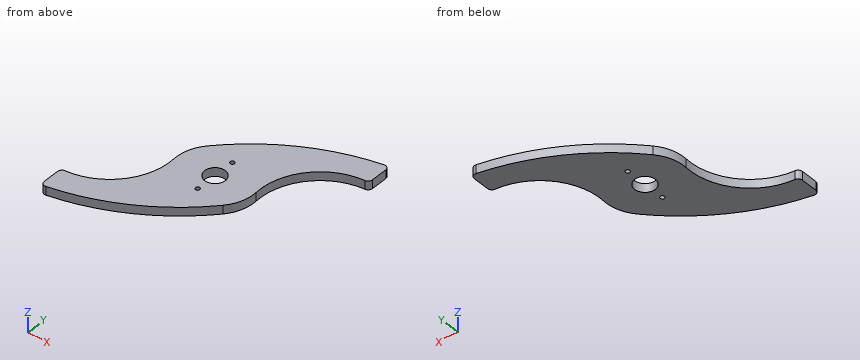
from build123d import *

# Parameters (mm, degrees)
SKETCH1_R           = 45
SKETCH1_R_2         = 12
BOSS_EXTRUDE1_DEPTH = 10
BOSS_EXTRUDE3_START = -10
BOSS_EXTRUDE3_DEPTH = 10
FILLET2_R           = 5
SKETCH3_R           = 2.5
CUT_EXTRUDE1_DEPTH  = 159.845357518


with BuildPart() as part:
    # Sketch1 → Boss-Extrude1 (new body)
    with BuildSketch(Plane.XY):
        Circle(SKETCH1_R)
        Circle(SKETCH1_R_2, mode=Mode.SUBTRACT)
    extrude(amount=BOSS_EXTRUDE1_DEPTH)

    # Sketch2 → Boss-Extrude3 (add)
    with BuildSketch(Plane.XY.offset(10).offset(BOSS_EXTRUDE3_START)):
        with BuildLine():
            ThreePointArc((33.436200174, -30.116781334), (-14.286491123, -42.671960013), (-44.829498519, -3.91357414))
            ThreePointArc((-44.829498519, -3.91357414), (-63.106761283, -57.457908747), (-115, -80))
            Line((-115, -80), (-115, -110))
            ThreePointArc((-115, -110), (-33.84606429, -82.946317595), (33.436200174, -30.116781334))
        make_face()
        with BuildLine():
            Line((115, 80), (115, 110))
            ThreePointArc((115, 110), (33.84606429, 82.946317595), (-33.436200174, 30.116781334))
            ThreePointArc((-33.436200174, 30.116781334), (14.286491123, 42.671960013), (44.829498519, 3.91357414))
            ThreePointArc((44.829498519, 3.91357414), (63.106761283, 57.457908747), (115, 80))
        make_face()
    extrude(amount=BOSS_EXTRUDE3_DEPTH)

    # Fillet2
    fillet2_edges = [part.edges().sort_by_distance(p)[0] for p in [
        (-115, -110, 5),
        (-115, -80, 5),
        (115, 80, 5),
        (115, 110, 5),
    ]]
    fillet(fillet2_edges, radius=FILLET2_R)

    # Sketch3 → Cut-Extrude1 (cut, through all)
    with BuildSketch(Plane.XY.offset(10)):
        with Locations((0, 25)):
            Circle(SKETCH3_R)
        with Locations((0, -25)):
            Circle(SKETCH3_R)
    extrude(amount=-CUT_EXTRUDE1_DEPTH, mode=Mode.SUBTRACT)


solid = part.part
Geometry: final body of the model. Coordinates: model frame, mm. Give positions to 0.01 mm unless a question says otherwise; leave off trailing zeros. Write each loop counter-clockwise with the first axis right and the second up, starting at its lowest first coordinate (ties: lowest second). Pieces come first, ordered by that corner, then holes. Notation, with made-up numbers: (55.5, -34) - (100.5, -34) arc R22 cw to (100.5, -13) - close; hole circle Ø11 at (-16, 59). An arc over 180 degrees is marked (long way). Return JSON: item names as keys, results as strings. Group by question number.
1) First-contact query: P1, Ø1, axis at y = 13.5, z = 5.5, coming from the -X side; P2, Ø2, axis at x = 62, z = 6.5, coming from the +Y side; P3, Ø1.5, axis at x = 73, z = 6, coming from the -Y side; P4, Ø4, axis at x = 0, y = -25, coming from the +Z side. Flat tips, straight axial feed; report the tip coordinate or a pass-through.
2) Section B-B on z = 5. Return the cut outline in (x, y).
3) Section D-D on y = -70.5. Return the cut outline in (x, z).
4) Line query: line 1 (Y direction, x = 0, z = 6.5); line 2 (Y direction, x = 9.5, z = 7.25); line 3 (X direction, y = 5, z = 0.5). Output: solid intervals per line, ascending.
5) Section A-A on y = 0. Return the cut outline in (x, z).
6) Section C-C on x = -36. Return the cut outline in (y, z).
Filled in:
{
 "1": {"P1": "stops at x = -43.08", "P2": "stops at y = 96.3", "P3": "stops at y = 65.76", "P4": "passes through"},
 "2": {"outline": "(-115, -104.12) arc R5 ccw to (-109.14, -109.04) arc R250 ccw to (33.44, -30.12) arc R45 ccw to (44.83, 3.91) arc R70 cw to (110.3, 79.87) arc R5 ccw to (115, 84.86) - (115, 104.12) arc R5 ccw to (109.14, 109.04) arc R250 ccw to (-33.44, 30.12) arc R45 ccw to (-44.83, -3.91) arc R70 cw to (-110.3, -79.87) arc R5 ccw to (-115, -84.86) - close; hole circle Ø24 at (0, 0); hole circle Ø5 at (0, -25); hole circle Ø5 at (0, 25)"},
 "3": {"outline": "(-79.35, 0) - (-13.18, 0) - (-13.18, 10) - (-79.35, 10) - close"},
 "4": {"line 1": "y = -61.04 to -27.5, -22.5 to -12, 12 to 22.5, 27.5 to 61.04", "line 2": "y = -53.36 to -7.33, 7.33 to 67.99", "line 3": "x = -44.72 to -10.91, 10.91 to 44.74"},
 "5": {"outline": "(-45, 0) - (-12, 0) - (-12, 10) - (-45, 10) - close; (12, 0) - (45, 0) - (45, 10) - (12, 10) - close"},
 "6": {"outline": "(-84.09, 0) - (27, 0) - (27, 10) - (-84.09, 10) - close"}
}
